from build123d import *

# Parameters (mm, degrees)
SKETCH1_R           = 1.0795
BOSS_EXTRUDE1_DEPTH = 0.8001
SKETCH2_R           = 3.81
BOSS_EXTRUDE2_DEPTH = 3.175
FILLET1_R           = 2.54


with BuildPart() as part:
    # Sketch1 → Boss-Extrude1 (new body, symmetric)
    with BuildSketch(Plane(origin=(0, 0, 0), x_dir=(1, 0, 0), z_dir=(0, 1, 0))):
        with BuildLine():
            Line((-13.4366, -7.0104), (13.4366, -7.0104))
            Line((13.4366, -7.0104), (13.4366, -8.1661))
            ThreePointArc((13.4366, -8.1661), (15.2781, -10.0076), (17.1196, -8.1661))
            Line((17.1196, -8.1661), (17.1196, -7.0104))
            Line((17.1196, -7.0104), (17.1196, 7.0104))
            Line((17.1196, 7.0104), (17.1196, 8.1661))
            ThreePointArc((17.1196, 8.1661), (15.2781, 10.0076), (13.4366, 8.1661))
            Line((13.4366, 8.1661), (13.4366, 7.0104))
            Line((13.4366, 7.0104), (-13.4366, 7.0104))
            Line((-13.4366, 7.0104), (-13.4366, 8.1661))
            ThreePointArc((-13.4366, 8.1661), (-15.2781, 10.0076), (-17.1196, 8.1661))
            Line((-17.1196, 8.1661), (-17.1196, 7.0104))
            Line((-17.1196, 7.0104), (-17.1196, -7.0104))
            Line((-17.1196, -7.0104), (-17.1196, -8.1661))
            ThreePointArc((-17.1196, -8.1661), (-15.2781, -10.0076), (-13.4366, -8.1661))
            Line((-13.4366, -8.1661), (-13.4366, -7.0104))
        make_face()
        with Locations((-15.2781, 8.1661)):
            Circle(SKETCH1_R, mode=Mode.SUBTRACT)
        with Locations((-15.2781, -8.1661)):
            Circle(SKETCH1_R, mode=Mode.SUBTRACT)
        with Locations((15.2781, 8.1661)):
            Circle(SKETCH1_R, mode=Mode.SUBTRACT)
        with Locations((15.2781, -8.1661)):
            Circle(SKETCH1_R, mode=Mode.SUBTRACT)
    extrude(amount=BOSS_EXTRUDE1_DEPTH, both=True)

    # Sketch2 → Boss-Extrude2 (add)
    with BuildSketch(Plane(origin=(0, 0.8001, 0), x_dir=(1, 0, 0), z_dir=(0, 1, 0))):
        with Locations((6.0706, -1.8542)):
            Circle(SKETCH2_R)
    extrude(amount=BOSS_EXTRUDE2_DEPTH)

    # Fillet1
    fillet1_edges = [part.edges().sort_by_distance(p)[0] for p in [
        (2.2606, 3.9751, 1.8542),
    ]]
    fillet(fillet1_edges, radius=FILLET1_R)


solid = part.part
Verification items for the finished model (mm, model axes). A direction names the side the tool comes from. Coordinates: 2 decimals unless noted, no trailing zeros. Order: outer loops, then holes, each group sorted by start corner. A loop starts at its lowest first (then second) coordinate and runs counter-clockwise, first axis right, second up.
1. Sectioned sample at A-A, the plane y = -0.15. Record the cut outline in (x, z), and give its area (3 significant figures).
Results found:
outline: (-17.12, -8.17) arc R1.84 ccw to (-13.44, -8.17) - (-13.44, -7.01) - (13.44, -7.01) - (13.44, -8.17) arc R1.84 ccw to (17.12, -8.17) - (17.12, 8.17) arc R1.84 ccw to (13.44, 8.17) - (13.44, 7.01) - (-13.44, 7.01) - (-13.44, 8.17) arc R1.84 ccw to (-17.12, 8.17) - close; hole circle Ø2.16 at (-15.28, -8.17); hole circle Ø2.16 at (-15.28, 8.17); hole circle Ø2.16 at (15.28, -8.17); hole circle Ø2.16 at (15.28, 8.17)
area: 504 mm2
2. Set-up check for faces 1 (the face through (2.264, 1.113, 1.687)), 2 (the face through (-13.437, 0, -8)), 3 (the face through (13.437, 0, 8)): record each of +Z, -Z, +X, -X, +Y, -Y from which the full face is reachable in a straight line by a thin tool's end or side.
Results found:
face 1: +Y
face 2: -Z, +Y, -Y
face 3: +Z, +Y, -Y
3. Sectioned sample at D-D, the plane z = -3.75. Record the cut outline in (x, y).
Results found:
outline: (-17.12, -0.8) - (17.12, -0.8) - (17.12, 0.8) - (-17.12, 0.8) - close
4. Scan lines: line 1 (Y direction, x = 12.5, z = -3.5); line 2 (Z direction, x = 11, y = 0.2); line 3 (Y direction, x = 8, z = 0). Record each from-to range of solid material in increasing order.
Results found:
line 1: y = -0.8 to 0.8
line 2: z = -7.01 to 7.01
line 3: y = -0.8 to 3.55
5. Sectioned sample at B-B, the plane z = -8.5. Record the cut outline in (x, y).
Results found:
outline: (-17.09, -0.8) - (-16.3, -0.8) - (-16.3, 0.8) - (-17.09, 0.8) - close; (-14.25, -0.8) - (-13.47, -0.8) - (-13.47, 0.8) - (-14.25, 0.8) - close; (13.47, -0.8) - (14.25, -0.8) - (14.25, 0.8) - (13.47, 0.8) - close; (16.3, -0.8) - (17.09, -0.8) - (17.09, 0.8) - (16.3, 0.8) - close
6. Go/stop test with flat-tipped pins: pin 1 Ø1 at (x, y) = (7, 0) entering from +Z; pin 2 Ø3 at (x, z) = (-15.28, 8.17) entering from +Y; pin 3 Ø0.8 at (x, y) = (0, 0) entering from -Z. Record where each tip stops, or that it passes through.
Results found:
pin 1: stops at z = 7.01
pin 2: stops at y = 0.8
pin 3: stops at z = -7.01
7. Release check for a two-part mould opening along X. For faces 4 (the face through (17.12, 0, 0)), 5 (the face through (-15.319, 0.011, 10.007)), 6 (the face through (0, 0.8, 0)) record: +X half, -X half, draft (parallel to the pull), parting line (faces both ways), or undercut.
Results found:
face 4: +X half
face 5: undercut
face 6: draft
8. Sectioned sample at C-C, the plane x = -2. Record the cut outline in (y, z).
Results found:
outline: (-0.8, -7.01) - (0.8, -7.01) - (0.8, 7.01) - (-0.8, 7.01) - close
